Build history of the part. All positions in model axes, mm. A direction names the side the tool comes from. Give positions to 0.01 mm unless a question says otherwise; leave off trailing zeros. Loops run counter-clockwise (first coordinate to the right, second up) from the corner with the lowest first, then second, coordinate; pieces in that order, holes last. Notation, with made-up numbers: M -27,79.25 L 7,79.25 A24 ccw 7,103.25 Z; hole C 47.5,62 d5. An arc over 180 degrees is marked long. Answer as a JSON object with one key per item and string values. Group by question number.
1. Drop flat-ended pins along their axis: pin 1 Ø0.7 at (x, y) = (0.5, 2) entering from -Z; pin 2 Ø3 at (x, y) = (-1.5, 11.5) entering from -Z; pin 3 Ø2 at (y, z) = (12, 2) entering from +X; pin 4 Ø2 at (y, z) = (1.5, 0.5) entering from +X. Give the stop position or say it passes through.
2. Slice it at B-B (y = 3). List the corners of the cut face in (x, z).
3. Slice it at C-C (y = 6.75). List the corners of the cut face in (x, z), then the cut area to 3 significant figures.
4. 3-axis set-ups, long thin cutter, end or side, ignore diameter. For faces 1 (the face through (1.6, 3.1, 0.94)), 2 (the face through (-4.296, 2.62, -0.189)): which of +Z, -Z, +X, -X, +Y, -Y reach the whole face in a straight line?
5. Mould opens along X. For faces 3 (the face through (-0.54, 9.73, 2.44)), 4 (the face through (0, 14.8, 0)), 5 (the face through (-1.872, 0.143, 1.058)), 6 (the face through (-1.74, 1.61, -0.99)) say: released by +X, released by -X, zero draft, split by the parting line, or undercut.
6. Drill centre lines: line 1 along Z through (x, y) = (2, 9.75); line 2 along X through (y, z) = (2.5, -1); line 3 along Y through (x, z) = (-0.75, 2.5). Where is each one in solid material? Low to high. Write a range as [from, to].
7. Slice it at A-A (x = 0). List the corners of the cut face in (y, z), then the cut area to 3 significant figures.
from build123d import *

# Parameters (mm, degrees)
SKETCH2_R           = 4.3
BOSS_EXTRUDE1_DEPTH = 4.8
SKETCH3_R           = 2.5
BOSS_EXTRUDE2_DEPTH = 10
CUT_EXTRUDE1_DEPTH  = 3.25
FILLET1_R           = 0.5


with BuildPart() as part:
    # Sketch2 → Boss-Extrude1 (new body)
    with BuildSketch(Plane(origin=(0, 0, 0), x_dir=(1, 0, 0), z_dir=(0, 1, 0))):
        Circle(SKETCH2_R)
    extrude(amount=BOSS_EXTRUDE1_DEPTH)

    # Sketch3 → Boss-Extrude2 (add)
    with BuildSketch(Plane(origin=(0, 4.8, 0), x_dir=(1, 0, 0), z_dir=(0, 1, 0))):
        Circle(SKETCH3_R)
    extrude(amount=BOSS_EXTRUDE2_DEPTH)

    # Sketch5 → Cut-Extrude1 (cut)
    with BuildSketch(Plane.XZ):
        Polygon((-1.154700538, 2), (-2.309401077, 0), (-1.154700538, -2), (1.154700538, -2), (2.309401077, 0), (1.154700538, 2), align=None)
    extrude(amount=-CUT_EXTRUDE1_DEPTH, mode=Mode.SUBTRACT)

    # Fillet1
    fillet1_edges = [part.edges().sort_by_distance(p)[0] for p in [
        (0, 3.25, 2),
        (1.732050808, 3.25, 1),
        (1.732050808, 3.25, -1),
        (0, 3.25, -2),
        (-1.732050808, 3.25, -1),
        (-1.732050808, 3.25, 1),
        (0, 0, 2),
        (-1.732050808, 0, 1),
        (-1.732050808, 0, -1),
        (0, 0, -2),
        (1.732050808, 0, -1),
        (1.732050808, 0, 1),
        (-4.3, 0, 0),
    ]]
    fillet(fillet1_edges, radius=FILLET1_R)


solid = part.part
Established:
{
 "1": {"pin 1": "stops at z = -4.3", "pin 2": "stops at z = -2.5", "pin 3": "stops at x = 2.29", "pin 4": "stops at x = 4.3"},
 "2": {"outline": "C 0,0 d8.6; hole M -2.23,0 L -1.12,-1.93 L 1.12,-1.93 L 2.23,0 L 1.12,1.93 L -1.12,1.93 Z"},
 "3": {"outline": "C 0,0 d5", "area": "19.6 mm^2"},
 "4": {"face 1": "-Y", "face 2": "+Y, -Y"},
 "5": {"face 3": "split by the parting line", "face 4": "zero draft", "face 5": "undercut", "face 6": "undercut"},
 "6": {"line 1": "z = [-1.5, 1.5]", "line 2": "x = [-4.18, -1.73], [1.73, 4.18]", "line 3": "y = [0, 4.8]"},
 "7": {"outline": "M 0,-3.8 A0.5 ccw 0.5,-4.3 L 4.8,-4.3 L 4.8,-2.5 L 14.8,-2.5 L 14.8,2.5 L 4.8,2.5 L 4.8,4.3 L 0.5,4.3 A0.5 ccw 0,3.8 L 0,2.5 A0.5 ccw 0.5,2 L 2.75,2 A0.5 cw 3.25,1.5 L 3.25,-1.5 A0.5 cw 2.75,-2 L 0.5,-2 A0.5 ccw 0,-2.5 Z", "area": "78.2 mm^2"}
}
